Input: part model. Units: mm. Frame: model coordinates. A direction names the side the tool comes from. Coordinates: 2 decimals unless noted, no trailing zeros. Write each loop counter-clockwise with the first axis right and the second up, starting at its lowest first coordinate (ties: lowest second). Pieces come first, ordered by that corner, then holes. Notation, with made-up numbers: M 13.5,73.25 L 28.5,73.25 A24 cw 28.5,102.25 Z; hole C -19,24 d6. An arc over 180 degrees is marked long. Write each question's results on one line, items separated by ' | '. Start each with the question number.
1. Set-up query: faces 1 (the flat face through (0, -10, 102.6)), 2 (the flat face through (-76.005, -10, 41)), 3 (the flat face through (1, -10, 15)), 4 (the cylindrical face through (72.05, -10.14, 98.86)). Return all of +Z, -Z, +X, -X, +Y, -Y with unobstructed straight access to the full face (end or side cutting, diameter ignored); none if empty.
2. Section query D-D, the plane z = 79. Output: boundary loops of the cut face in (x, y).
3. Ray query, probe 1 along Z at (x, y) = (-63, -9.5); probe 2 along X at (y, z) = (-10.75, 12.5); probe 3 along Z at (x, y) = (-68.5, -8.5). Return the intervals inside material, ascending.
4. Section query B-B, the plane x = -81.5. Output: boundary loops of the cut face in (y, z), and give its area (3 significant figures).
5. Pull-direction query (X, two-part tool) for faces 5 (the cylindrical face through (-93.44, -9.86, -36.57)), 6 (the flat face through (75.995, -10, 40)), 7 (the flat face through (-48.005, -10, 0)); classes: +X half, -X half, draft (parallel to the pull), parting line (faces both ways), or undercut.
6. Section query A-A, the plane x = 0. Output: boundary loops of the cut face in (y, z), and give its area (3 significant figures).
7. Section query C-C, the plane y = -16. Count the separate pieces of the cut face and the enclosed holes in it, and give its area (3 significant figures).
8. First-contact query: pin 1 (2 mm diameter, centred on x = -0.5, y = -3.5, fed in from +Z); pin 2 (2 mm diameter, centred on y = -6.5, z = 34, fed in from -X); pin 3 (4.5 mm diameter, centred on x = -57, y = -11.5, fed in from +Z). Flat tips, straight axial feed; report the tip coordinate or a pass-through.
```python
from build123d import *

# Parameters (mm, degrees)
F0_R        = 15
F0_R_2      = 1.6
F1_DEPTH    = 20
F2_R        = 11.6045153918
F3_DEPTH    = 20
F4_T1_DEPTH = 334.7254047122
F6_R        = 13.1169251871
F7_T1_DEPTH = 119.353153646
F7_T3_DEPTH = 204.1085089788


# Not quite as in the source:
# - a fillet or chamfer that OpenCascade refuses, or shapes differently, is made with other operations: its cross-section is extruded or revolved along the edge and cut away or added


with BuildPart() as f1:
    # F0 (on Front) → F1 (new body)
    with BuildSketch(Plane.XZ):
        Polygon((-54.1030839086, 102.6), (-76.0052064898, 102.6), (-76.0052064898, -8.4487323015), (-76.0052064898, -58.9213789776), (-76.0052064898, -97.4), (75.9947935102, -97.4), (75.9947935102, -58.9213789776), (75.9947935102, -8.4487323015), (75.9947935102, 102.6), (54.0926709289, 102.6), (3.7848638975, 102.6), (-0.0052064898, 102.6), (-3.7952768771, 102.6), align=None)
        with Locations((0, -60)):
            Circle(F0_R, mode=Mode.SUBTRACT)
        Polygon((-48.0052064898, 15), (-0.0052064898, 15), (50.9947935102, 15), (63.2902167228, 1.058300535), (64.2235500655, 0), (63.2902167424, -1.0583005129), (50.9947935102, -15), (-48.0052064898, -15), (-61.2339630452, 0), align=None, mode=Mode.SUBTRACT)
        with Locations((-68.4052064898, 60)):
            Circle(F0_R_2, mode=Mode.SUBTRACT)
        with Locations((-62.4052064898, 60)):
            Circle(F0_R_2, mode=Mode.SUBTRACT)
        with Locations((-56.4052064898, 60)):
            Circle(F0_R_2, mode=Mode.SUBTRACT)
        with Locations((-68.4052064898, 89)):
            Circle(F0_R_2, mode=Mode.SUBTRACT)
        with Locations((-62.4052064898, 89)):
            Circle(F0_R_2, mode=Mode.SUBTRACT)
        with Locations((-56.4052064898, 89)):
            Circle(F0_R_2, mode=Mode.SUBTRACT)
        with Locations((56.3947935102, 60)):
            Circle(F0_R_2, mode=Mode.SUBTRACT)
        with Locations((62.3947935102, 60)):
            Circle(F0_R_2, mode=Mode.SUBTRACT)
        with Locations((68.3947935102, 60)):
            Circle(F0_R_2, mode=Mode.SUBTRACT)
        with Locations((56.3947935102, 89)):
            Circle(F0_R_2, mode=Mode.SUBTRACT)
        with Locations((62.3947935102, 89)):
            Circle(F0_R_2, mode=Mode.SUBTRACT)
        with Locations((68.3947935102, 89)):
            Circle(F0_R_2, mode=Mode.SUBTRACT)
        Polygon((-77.668659389, 119.0051808953), (-54.1030839086, 102.6), (-3.7952768771, 102.6), (-65.412312746, 145.4675197601), (-108.1871464849, 109.1671809554), align=None)
        Polygon((-76.0052064898, -58.9213789776), (-76.0052064898, -8.4487323015), (-103.1352177745, -45.4250201583), (-90.5148283129, -43.2038009167), (-105.0179273372, -79.8825249076), align=None)
        Polygon((65.4018997664, 145.4675197601), (3.7848638975, 102.6), (54.0926709289, 102.6), (77.6582464094, 119.0051808953), (108.1767335052, 109.1671809554), align=None)
        Polygon((75.9947935102, -8.4487323015), (75.9947935102, -58.9213789776), (105.0075143576, -79.8825249076), (90.5044153333, -43.2038009167), (103.1248047948, -45.4250201583), align=None)
        with BuildLine():
            Line((63.2902167228, 1.058300535), (50.9947935102, 15))
            Line((50.9947935102, 15), (50.9947935102, -15))
            Line((50.9947935102, -15), (63.2902167424, -1.0583005129))
            ThreePointArc((63.2902167424, -1.0583005129), (60.4902167322, -1.48e-08), (63.2902167228, 1.058300535))
        make_face()
        Polygon((-48.0052064898, -15), (-48.0052064898, 15), (-61.2339630452, 0), align=None)
        with Locations((-58.9281324463, 0)):
            Circle(F0_R_2, mode=Mode.SUBTRACT)
    extrude(amount=F1_DEPTH)

    # F2
    f2_edges = [f1.edges().sort_by_distance(p)[0] for p in [
        (-76.005206, -10, 102.6),
        (-76.005206, -10, -97.4),
        (75.994794, -10, -97.4),
        (75.994794, -10, 102.6),
    ]]
    fillet(f2_edges, radius=F2_R)

    # F0 (on Front) → F3 (join)
    with BuildSketch(Plane.XZ):
        Polygon((-54.1030839086, 102.6), (-76.0052064898, 102.6), (-76.0052064898, -8.4487323015), (-76.0052064898, -58.9213789776), (-76.0052064898, -97.4), (75.9947935102, -97.4), (75.9947935102, -58.9213789776), (75.9947935102, -8.4487323015), (75.9947935102, 102.6), (54.0926709289, 102.6), (3.7848638975, 102.6), (-0.0052064898, 102.6), (-3.7952768771, 102.6), align=None)
        with Locations((0, -60)):
            Circle(F0_R, mode=Mode.SUBTRACT)
        Polygon((-48.0052064898, 15), (-0.0052064898, 15), (50.9947935102, 15), (63.2902167228, 1.058300535), (64.2235500655, 0), (63.2902167424, -1.0583005129), (50.9947935102, -15), (-48.0052064898, -15), (-61.2339630452, 0), align=None, mode=Mode.SUBTRACT)
        with Locations((-68.4052064898, 60)):
            Circle(F0_R_2, mode=Mode.SUBTRACT)
        with Locations((-62.4052064898, 60)):
            Circle(F0_R_2, mode=Mode.SUBTRACT)
        with Locations((-56.4052064898, 60)):
            Circle(F0_R_2, mode=Mode.SUBTRACT)
        with Locations((-68.4052064898, 89)):
            Circle(F0_R_2, mode=Mode.SUBTRACT)
        with Locations((-62.4052064898, 89)):
            Circle(F0_R_2, mode=Mode.SUBTRACT)
        with Locations((-56.4052064898, 89)):
            Circle(F0_R_2, mode=Mode.SUBTRACT)
        with Locations((56.3947935102, 60)):
            Circle(F0_R_2, mode=Mode.SUBTRACT)
        with Locations((62.3947935102, 60)):
            Circle(F0_R_2, mode=Mode.SUBTRACT)
        with Locations((68.3947935102, 60)):
            Circle(F0_R_2, mode=Mode.SUBTRACT)
        with Locations((56.3947935102, 89)):
            Circle(F0_R_2, mode=Mode.SUBTRACT)
        with Locations((62.3947935102, 89)):
            Circle(F0_R_2, mode=Mode.SUBTRACT)
        with Locations((68.3947935102, 89)):
            Circle(F0_R_2, mode=Mode.SUBTRACT)
        Polygon((-77.668659389, 119.0051808953), (-54.1030839086, 102.6), (-3.7952768771, 102.6), (-65.412312746, 145.4675197601), (-108.1871464849, 109.1671809554), align=None)
        Polygon((-76.0052064898, -58.9213789776), (-76.0052064898, -8.4487323015), (-103.1352177745, -45.4250201583), (-90.5148283129, -43.2038009167), (-105.0179273372, -79.8825249076), align=None)
        Polygon((65.4018997664, 145.4675197601), (3.7848638975, 102.6), (54.0926709289, 102.6), (77.6582464094, 119.0051808953), (108.1767335052, 109.1671809554), align=None)
        Polygon((75.9947935102, -8.4487323015), (75.9947935102, -58.9213789776), (105.0075143576, -79.8825249076), (90.5044153333, -43.2038009167), (103.1248047948, -45.4250201583), align=None)
        Polygon((-48.0052064898, -15), (-48.0052064898, 15), (-61.2339630452, 0), align=None)
        with Locations((-58.9281324463, 0)):
            Circle(F0_R_2, mode=Mode.SUBTRACT)
        with BuildLine():
            Line((63.2902167228, 1.058300535), (50.9947935102, 15))
            Line((50.9947935102, 15), (50.9947935102, -15))
            Line((50.9947935102, -15), (63.2902167424, -1.0583005129))
            ThreePointArc((63.2902167424, -1.0583005129), (60.4902167322, -1.48e-08), (63.2902167228, 1.058300535))
        make_face()
    extrude(amount=F3_DEPTH)

    # F4: fillet of radius 70.723525766 on 2 edges, made by hand

    # F4_s2 → F4_t1 (cut)
    with BuildSketch(Plane.XZ.offset(-157.3627023561)):
        with BuildLine():
            ThreePointArc((-76.0052064898, -58.9213789776), (-49.9474116045, -87.018376956), (-13.0601255474, -97.4))
            Line((-13.0601255474, -97.4), (-76.0052064898, -97.4))
            Line((-76.0052064898, -97.4), (-76.0052064898, -58.9213789776))
        make_face()
        with BuildLine():
            ThreePointArc((13.0497125677, -97.4), (49.9369986248, -87.018376956), (75.9947935102, -58.9213789776))
            Line((75.9947935102, -58.9213789776), (75.9947935102, -97.4))
            Line((75.9947935102, -97.4), (13.0497125677, -97.4))
        make_face()
    extrude(amount=F4_T1_DEPTH, mode=Mode.SUBTRACT)

    # F6
    f6_edges = [f1.edges().sort_by_distance(p)[0] for p in [
        (75.994794, -10, 102.6),
        (-76.005206, -10, 102.6),
    ]]
    fillet(f6_edges, radius=F6_R)

    # F7: fillet of radius 10.7873299095 on 4 edges, made by hand

    # F7_s2 → F7_t1 (cut)
    with BuildSketch(Plane.XZ.offset(-49.676576823)):
        with BuildLine():
            ThreePointArc((91.3700727829, -29.4041512397), (93.4388619061, -36.4609035493), (90.5044153333, -43.2038009167))
            Line((90.5044153333, -43.2038009167), (103.1248047948, -45.4250201583))
            Line((103.1248047948, -45.4250201583), (91.3700727829, -29.4041512397))
        make_face()
        with BuildLine():
            ThreePointArc((-90.5148283129, -43.2038009167), (-93.4492748858, -36.4609035493), (-91.3804857626, -29.4041512397))
            Line((-91.3804857626, -29.4041512397), (-103.1352177745, -45.4250201583))
            Line((-103.1352177745, -45.4250201583), (-90.5148283129, -43.2038009167))
        make_face()
    extrude(amount=F7_T1_DEPTH, mode=Mode.SUBTRACT)

    # F7_s4 → F7_t3 (cut)
    with BuildSketch(Plane.XZ.offset(-92.0542544894)):
        with BuildLine():
            ThreePointArc((-76.0052064898, -58.9213789776), (-88.4725874625, -57.7926608942), (-91.4783185714, -45.6404934608))
            Line((-91.4783185714, -45.6404934608), (-105.0179273372, -79.8825249076))
            Line((-105.0179273372, -79.8825249076), (-76.0052064898, -58.9213789776))
        make_face()
        with BuildLine():
            ThreePointArc((91.4679055918, -45.6404934608), (88.4621744828, -57.7926608942), (75.9947935102, -58.9213789776))
            Line((75.9947935102, -58.9213789776), (105.0075143576, -79.8825249076))
            Line((105.0075143576, -79.8825249076), (91.4679055918, -45.6404934608))
        make_face()
    extrude(amount=F7_T3_DEPTH, mode=Mode.SUBTRACT)


solid = f1.part
```
Answer:
1) face 1: +Z, +Y, -Y | face 2: -X, +Y, -Y | face 3: +Y, -Y | face 4: +X, +Y, -Y
2) outline: M -76.01,-20 L 75.99,-20 L 75.99,0 L -76.01,0 Z
3) probe 1: -76.75 to 58.51, 61.49 to 87.51, 90.49 to 102.6, 108.79 to 143.79 | probe 2: -76.01 to -48.01, 50.99 to 75.99 | probe 3: -70.59 to 58.4, 61.6 to 87.4, 90.6 to 101.34, 112.62 to 142.85
4) outline: M -20,-60.39 L 0,-60.39 L 0,-15.94 L -20,-15.94 Z; M -20,117.77 L 0,117.77 L 0,131.81 L -20,131.81 Z | area: 1,170 mm^2
5) face 5: -X half | face 6: +X half | face 7: undercut
6) outline: M -20,-97.4 L 0,-97.4 L 0,-75 L -20,-75 Z; M -20,-45 L 0,-45 L 0,-15 L -20,-15 Z; M -20,15 L 0,15 L 0,102.6 L -20,102.6 Z | area: 2,800 mm^2
7) separate pieces: 1 | enclosed holes: 16 | area: 30,100 mm^2
8) pin 1: z = 102.6 | pin 2: x = -76.01 | pin 3: z = 141.18
